CAD build for the part. Positions are in the model's coordinates, mm. Face numbers are marked on the shaded views. A direction names the side the tool comes from. Coordinates: 2 decimals unless noted, no trailing zeros. Order: outer loops, then holes, each group sorted by start corner. A loop starts at its lowest first (then second) coordinate and runs counter-clockwise, first axis right, second up. Notation, with made-up numbers: (33.25, 26.5) - (75.25, 26.5) arc R11 ccw to (75.25, 41.5) - close; hole circle Ø7 at (11.5, 75). An arc over 180 degrees is marked (long way). Use one line per item in the form item = value.
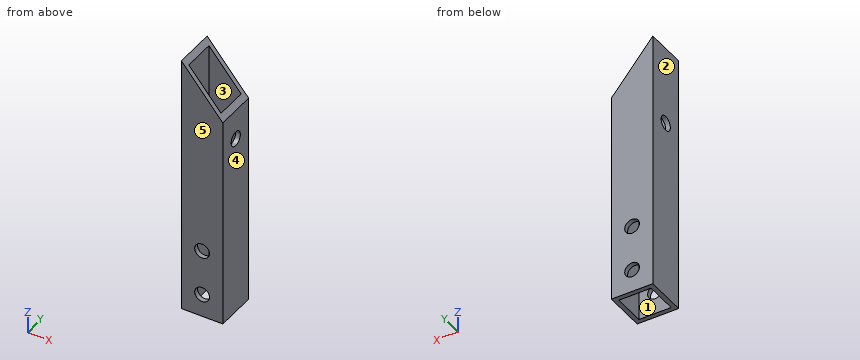
```python
from build123d import *

# Parameters (mm, degrees)
SKETCH_1_W          = 9
SKETCH_1_H          = 9
SKETCH_1_W_2        = 7
SKETCH_1_H_2        = 7
EXTRUDE_1_DEPTH     = 70
SKETCH_2_R          = 1.6
CUT_EXTRUDE_1_DEPTH = 50
CUT_EXTRUDE_2_DEPTH = 10
SKETCH_4_W          = 9
SKETCH_4_H          = 13
CUT_EXTRUDE_3_DEPTH = 10
SKETCH_5_R          = 1.6
CUT_EXTRUDE_4_DEPTH = 400


with BuildPart() as part:
    # ｽｹｯﾁ1 → ﾎﾞｽ - 押し出し1 (new body)
    with BuildSketch(Plane.XY):
        Rectangle(SKETCH_1_W, SKETCH_1_H)
        Rectangle(SKETCH_1_W_2, SKETCH_1_H_2, mode=Mode.SUBTRACT)
    extrude(amount=EXTRUDE_1_DEPTH)

    # ｽｹｯﾁ2 → ｶｯﾄ - 押し出し1 (cut)
    with BuildSketch(Plane(origin=(0, 4.5, 0), x_dir=(1, 0, 0), z_dir=(0, 1, 0))):
        with Locations((0, -5)):
            Circle(SKETCH_2_R)
        with Locations((0, -15)):
            Circle(SKETCH_2_R)
    extrude(amount=-CUT_EXTRUDE_1_DEPTH, mode=Mode.SUBTRACT)

    # ｽｹｯﾁ3 → ｶｯﾄ - 押し出し2 (cut)
    with BuildSketch(Plane(origin=(0, 4.5, 0), x_dir=(1, 0, 0), z_dir=(0, 1, 0))):
        Polygon((4.5, -46.274217667), (-4.5, -57), (4.5, -57), align=None)
    extrude(amount=-CUT_EXTRUDE_2_DEPTH, mode=Mode.SUBTRACT)

    # ｽｹｯﾁ4 → ｶｯﾄ - 押し出し3 (cut)
    with BuildSketch(Plane(origin=(0, 4.5, 0), x_dir=(1, 0, 0), z_dir=(0, 1, 0))):
        with Locations((0, -63.5)):
            Rectangle(SKETCH_4_W, SKETCH_4_H)
    extrude(amount=-CUT_EXTRUDE_3_DEPTH, mode=Mode.SUBTRACT)

    # ｽｹｯﾁ5 → ｶｯﾄ - 押し出し4 (cut)
    with BuildSketch(Plane(origin=(4.5, 0, 0), x_dir=(0, 0, -1), z_dir=(1, 0, 0))):
        with Locations((-39.774217667, 0)):
            Circle(SKETCH_5_R)
    extrude(amount=-CUT_EXTRUDE_4_DEPTH, mode=Mode.SUBTRACT)


solid = part.part
```
Item 1: Cut at A-A, the plane y = 0. Write the cut outline in (x, z), plus the area to 3 significant figures.
Derived:
outline = (-4.5, 0) - (-3.5, 0) - (-3.5, 38.17) - (-4.5, 38.17) - close; (-4.5, 41.37) - (-3.5, 41.37) - (-3.5, 55.81) - (-4.5, 57) - close; (3.5, 0) - (4.5, 0) - (4.5, 38.17) - (3.5, 38.17) - close; (3.5, 41.37) - (4.5, 41.37) - (4.5, 46.27) - (3.5, 47.47) - close
area = 96.9 mm²
Item 2: Two-plate mould, pull along X, no slides. Class the marked faces 3, 4 and 5: +X half, -X half, draft (parallel to the pull), parting line (faces both ways), or undercut.
Derived:
face_3 = undercut
face_4 = +X half
face_5 = draft
Item 3: Drill centre lines: line 1 (X direction, y = -4.2, z = 15); line 2 (X direction, y = -2.5, z = 40.5); line 3 (Z direction, x = 0.25, y = 4.25). Where is each one in solid material? Low to high. Write a range as [from, to].
Derived:
line_1 = [-4.5, -1.6], [1.6, 4.5]
line_2 = [-4.5, -3.5], [3.5, 4.5]
line_3 = [0, 3.42], [6.58, 13.42], [16.58, 51.34]
Item 4: Cut at D-D, the plane x = -2.5. Write the cut outline in (y, z).
Derived:
outline = (-4.5, 0) - (-3.5, 0) - (-3.5, 54.62) - (-4.5, 54.62) - close; (3.5, 0) - (4.5, 0) - (4.5, 54.62) - (3.5, 54.62) - close
Item 5: Drop a flat-ended pin along its axis: pin 1 (5 mm diameter, centred on x = 2, y = -3, fed in from +Z). Give the stop position or say it passes through.
Derived:
pin_1 = 52.17
Item 6: Cut at C-C, the plane y = 2.5. Write the cut outline in (x, z).
Derived:
outline = (-4.5, 0) - (-3.5, 0) - (-3.5, 55.81) - (-4.5, 57) - close; (3.5, 0) - (4.5, 0) - (4.5, 46.27) - (3.5, 47.47) - close
Item 7: Cut at B-B, the plane z = 15. Write the cut outline in (x, y).
Derived:
outline = (-4.5, -4.5) - (-1.6, -4.5) - (-1.6, -3.5) - (-3.5, -3.5) - (-3.5, 3.5) - (-1.6, 3.5) - (-1.6, 4.5) - (-4.5, 4.5) - close; (1.6, -4.5) - (4.5, -4.5) - (4.5, 4.5) - (1.6, 4.5) - (1.6, 3.5) - (3.5, 3.5) - (3.5, -3.5) - (1.6, -3.5) - close
Item 8: 3-axis set-ups, long thin cutter, end or side, ignore diameter. For the marked faces 1 and 2: which of +Z, -Z, +X, -X, +Y, -Y reach the whole face in a straight line?
Derived:
face_1 = +Z, -Z
face_2 = +Z, -Z, -X, +Y, -Y
